Geometry: final body of the model. Coordinates: model frame, mm. A direction names the side the tool comes from. Give positions to 0.01 mm unless a question says otherwise; leave off trailing zeros. Order: outer loops, then holes, each group sorted by start corner. A loop starts at its lowest first (then second) coordinate and runs counter-clockwise, first axis right, second up. Notation, with made-up numbers: (-22, 54.25) -> (25, 54.25) arc R34 ccw to (25, 87.25) -> close; hole circle Ø6 at (-21, 44.5). An arc over 180 degrees is marked (long way). Write item = value, one per line.
Autodesk Inventor part; units mm, degrees
ref_plane "YZ Plane" through (0, 0, 0) normal (1, 0, 0) x (0, 1, 0)
ref_plane "XZ Plane" through (0, 0, 0) normal (0, 1, 0) x (-1, 0, 0)
ref_plane "XY Plane" through (0, 0, 0) normal (0, 0, 1) x (1, 0, 0)
sketch "스케치1" plane through (0, 0, 0) normal (0, 0, 1) x (1, 0, 0)
  line L0 (0, 0) -> (142, 0)
  line L1 (142, 0) -> (142, -30)
  line L2 (142, -30) -> (0, -30)
  line L3 (0, -30) -> (0, 0)
  line L4 (2, -2) -> (28, -2)
  line L5 (28, -2) -> (28, -28)
  line L6 (28, -28) -> (2, -28)
  line L7 (2, -28) -> (2, -2)
  line L8 (56, -2) -> (56, -28)
  line L9 (30, -2) -> (56, -2)
  line L10 (30, -28) -> (30, -2)
  line L11 (56, -28) -> (30, -28)
  line L12 (84, -2) -> (84, -28)
  line L13 (58, -2) -> (84, -2)
  line L14 (58, -28) -> (58, -2)
  line L15 (84, -28) -> (58, -28)
  line L16 (112, -2) -> (112, -28)
  line L17 (86, -2) -> (112, -2)
  line L18 (86, -28) -> (86, -2)
  line L19 (112, -28) -> (86, -28)
  line L20 (140, -2) -> (140, -28)
  line L21 (114, -2) -> (140, -2)
  line L22 (114, -28) -> (114, -2)
  line L23 (140, -28) -> (114, -28)
  dimension "d0" = 142
  dimension "d1" = 30
  dimension "d2" = 2
  dimension "d3" = 2
  dimension "d4" = 26
  dimension "d5" = 26
  dimension "d8" = 28
extrude "돌출1" add sketch "스케치1" along normal blind 4
sketch "스케치2" plane through (0, 0, 4) normal (0, 0, 1) x (1, 0, 0)
  line L0 (0, -30) -> (142, -30)
  line L1 (142, -30) -> (142, 0)
  line L2 (142, 0) -> (0, 0)
  line L3 (0, 0) -> (0, -30)
  line L4 (140, -2) -> (140, -28)
  line L5 (140, -28) -> (114, -28)
  line L6 (114, -28) -> (114, -2)
  line L7 (114, -2) -> (140, -2)
  line L8 (112, -2) -> (112, -28)
  line L9 (112, -28) -> (86, -28)
  line L10 (86, -28) -> (86, -2)
  line L11 (86, -2) -> (112, -2)
  line L12 (84, -2) -> (84, -28)
  line L13 (84, -28) -> (58, -28)
  line L14 (58, -28) -> (58, -2)
  line L15 (58, -2) -> (84, -2)
  line L16 (56, -2) -> (56, -28)
  line L17 (56, -28) -> (30, -28)
  line L18 (30, -28) -> (30, -2)
  line L19 (30, -2) -> (56, -2)
  line L20 (2, -2) -> (28, -2)
  line L21 (28, -2) -> (28, -28)
  line L22 (28, -28) -> (2, -28)
  line L23 (2, -28) -> (2, -2)
extrude "돌출2" add sketch "스케치2" along normal blind 1 contours L3 L2 L1 L0 | L4 L5 L6 L7 | L8 L9 L10 L11 | L12 L13 L14 L15 | L16 L17 L18 L19 | L20 L21 L22 L23
fillet "모깎기1" radius 2 4 edges at (142, 0, 2.5) (142, -30, 2.5) (0, 0, 2.5) (0, -30, 2.5)
properties part number "t_pocket"
1) Section query A-A (z = 2.15). Output: boundary loops of the cut face in (x, y), plus the area to 3 significant figures.
Check sheet entries:
outline = (0, -28) arc R2 ccw to (2, -30) -> (140, -30) arc R2 ccw to (142, -28) -> (142, -2) arc R2 ccw to (140, 0) -> (2, 0) arc R2 ccw to (0, -2) -> close; hole (2, -28) -> (28, -28) -> (28, -2) -> (2, -2) -> close; hole (30, -28) -> (56, -28) -> (56, -2) -> (30, -2) -> close; hole (58, -28) -> (84, -28) -> (84, -2) -> (58, -2) -> close; hole (86, -28) -> (112, -28) -> (112, -2) -> (86, -2) -> close; hole (114, -28) -> (140, -28) -> (140, -2) -> (114, -2) -> close
area = 877 mm²
2) Section query B-B (x = 44). Output: boundary loops of the cut face in (y, z), plus the area to 3 significant figures.
Check sheet entries:
outline = (-30, 0) -> (-28, 0) -> (-28, 4) -> (-2, 4) -> (-2, 0) -> (0, 0) -> (0, 5) -> (-30, 5) -> close
area = 46.0 mm²
3) Mould query, pull axis X, two halves, no side actions, for faces 3 (the face through (72, -30, 2)), 4 (the face through (71, -2, 2)), 5 (the face through (0, -15, 2)). Classes: +X half, -X half, draft (parallel to the pull), parting line (faces both ways), or undercut.
Check sheet entries:
face_3 = draft
face_4 = undercut
face_5 = -X half
4) Line query: line 1 (X direction, y = -23.75, z = 1); line 2 (Y direction, x = 128.5, z = 0.5); line 3 (Z direction, x = 6, y = -18). Output: solid intervals per line, ascending. Write a range as from..to.
Check sheet entries:
line_1 = 0..2, 28..30, 56..58, 84..86, 112..114, 140..142
line_2 = -30..-28, -2..0
line_3 = 4..5
5) Reachability of faces 1 (the face through (70, -15, 5)), 2 (the face through (99, -2, 2)) from +Z, -Z, +X, -X, +Y, -Y: full face, straight path, thin tool, end or side. Return the list, or none.
Check sheet entries:
face_1 = +Z, +X, -X, +Y, -Y
face_2 = -Z
6) First-contact query: P1, Ø3, axis at x = 90, y = -16.5, coming from the -Z side. Flat tip, straight axial feed; report the tip coordinate or a pass-through.
Check sheet entries:
P1 = 4
7) Section query C-C (y = -20). Output: boundary loops of the cut face in (x, z), plus the area to 3 significant figures.
Check sheet entries:
outline = (0, 0) -> (2, 0) -> (2, 4) -> (28, 4) -> (28, 0) -> (30, 0) -> (30, 4) -> (56, 4) -> (56, 0) -> (58, 0) -> (58, 4) -> (84, 4) -> (84, 0) -> (86, 0) -> (86, 4) -> (112, 4) -> (112, 0) -> (114, 0) -> (114, 4) -> (140, 4) -> (140, 0) -> (142, 0) -> (142, 5) -> (0, 5) -> close
area = 190 mm²
